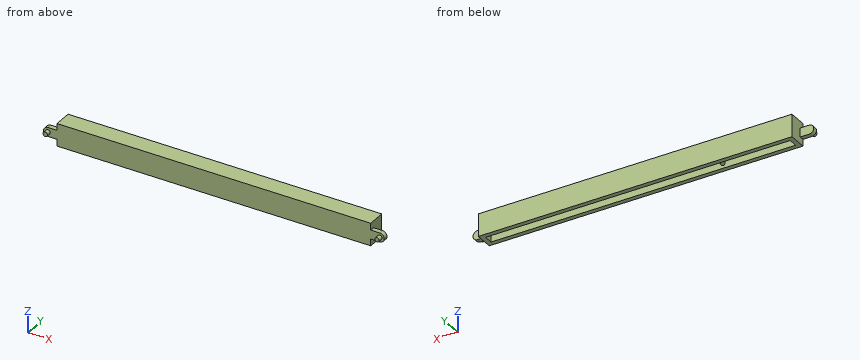
```python
from build123d import *

# Parameters (mm, degrees)
SKETCH1_W           = 67.6
SKETCH1_H           = 4
BASE_DEPTH          = 1
NOCK_DEPTH          = 1
WALLS_DEPTH         = 3
SKETCH4_W           = 69.6
SKETCH4_H           = 5
TOP_DEPTH           = 1
MOUNTINGTABS_DEPTH  = 1
SKETCH6_R           = 0.5
BOSS_EXTRUDE7_DEPTH = 1


with BuildPart() as part:
    # Sketch1 → Base (new body)
    with BuildSketch(Plane(origin=(0, 0, 0), x_dir=(1, 0, 0), z_dir=(0, 1, 0))):
        Rectangle(SKETCH1_W, SKETCH1_H)
    extrude(amount=BASE_DEPTH)

    # Sketch2 → nock (add)
    with BuildSketch(Plane(origin=(0, 1, 0), x_dir=(1, 0, 0), z_dir=(0, 1, 0))):
        with BuildLine():
            Line((-18.1, -2.5), (-18.1, 1))
            ThreePointArc((-18.1, 1), (-17.7, 1.4), (-17.3, 1))
            Line((-17.3, 1), (-17.3, -2.5))
            Line((-17.3, -2.5), (-18.1, -2.5))
        make_face()
    extrude(amount=NOCK_DEPTH)

    # Sketch3 → Walls (add)
    with BuildSketch(Plane(origin=(0, 0, 0), x_dir=(1, 0, 0), z_dir=(0, 1, 0))):
        Polygon((-33.8, 2), (-34.8, 2), (-34.8, -3), (34.8, -3), (34.8, 2), (33.8, 2), (33.8, -2), (-33.8, -2), align=None)
    extrude(amount=WALLS_DEPTH)

    # Sketch4 → Top (add)
    with BuildSketch(Plane(origin=(0, 3, 0), x_dir=(1, 0, 0), z_dir=(0, 1, 0))):
        with Locations((0, -0.5)):
            Rectangle(SKETCH4_W, SKETCH4_H)
    extrude(amount=TOP_DEPTH)

    # Sketch5 → MountingTabs (add)
    with BuildSketch(Plane(origin=(0, 0, 0), x_dir=(1, 0, 0), z_dir=(0, 1, 0))):
        with BuildLine():
            Line((-34.8, 0.5), (-34.8, -1.5))
            Line((-34.8, -1.5), (-36.8, -1.5))
            ThreePointArc((-36.8, -1.5), (-37.8, -0.5), (-36.8, 0.5))
            Line((-36.8, 0.5), (-34.8, 0.5))
        make_face()
        with BuildLine():
            Line((34.8, -1.5), (36.8, -1.5))
            ThreePointArc((36.8, -1.5), (37.8, -0.5), (36.8, 0.5))
            Line((36.8, 0.5), (34.8, 0.5))
            Line((34.8, 0.5), (34.8, -1.5))
        make_face()
    extrude(amount=MOUNTINGTABS_DEPTH)

    # Sketch6 → Boss-Extrude7 (add)
    with BuildSketch(Plane.XZ):
        with Locations(Location((-36.8, 0.5, 0), (0, 0, 270))):
            Circle(SKETCH6_R)
        with Locations(Location((36.8, 0.5, 0), (0, 0, 270))):
            Circle(SKETCH6_R)
    extrude(amount=BOSS_EXTRUDE7_DEPTH)


solid = part.part
```
Model file for the job. Use its own axes, mm. Coordinates: 2 decimals unless noted, no trailing zeros. Loops run counter-clockwise (first coordinate to the right, second up) from the corner with the lowest first, then second, coordinate; pieces in that order, holes last. Notation, with made-up numbers: (1.25, 14) - (46.25, 14) arc R21 ccw to (46.25, 30) - close; hole circle Ø5 at (-32, 30.5). An arc over 180 degrees is marked (long way). Write item = value, one per line. Start each with the question number.
Item 1: Drop flat-ended pins along their axis: pin 1 Ø0.6 at (y, z) = (2.5, 0.5) entering from +X; pin 2 Ø2 at (x, z) = (5.5, 2) entering from -Y; pin 3 Ø1 at (x, z) = (-35.5, 0.5) entering from +Y. Give the stop position or say it passes through.
Item 2: Saw through at A-A, the plane x = 1. List the corners of the cut face in (y, z), then the cut area to 3 significant figures.
Item 3: Wall check: probe 1 along X at (y, z) = (1.2, 0.2); probe 2 along Y at (x, z) = (10.5, -1); probe 3 along X at (y, z) = (2.35, 0.95). Give the ranges that are in metal, low to high. Write a range as [from, to].
Answers:
q1.pin_1 = 34.8
q1.pin_2 = 0
q1.pin_3 = 1
q2.outline = (0, -2) - (1, -2) - (1, 2) - (3, 2) - (3, -2) - (4, -2) - (4, 3) - (0, 3) - close
q2.area = 12.0 mm2
q3.probe_1 = [-34.8, -33.8], [-18.1, -17.3], [33.8, 34.8]
q3.probe_2 = [0, 1], [3, 4]
q3.probe_3 = [-34.8, -33.8], [33.8, 34.8]
